CAD build for the part. Positions are in the model's coordinates, mm. Give positions to 0.01 mm unless a question says otherwise; leave off trailing zeros. Loops run counter-clockwise (first coordinate to the right, second up) from the corner with the lowest first, then second, coordinate; pieces in that order, holes last. Notation, with made-up numbers: (27, 60.25) -> (83, 60.25) arc R13 cw to (83, 78.25) -> close; hole circle Ø9 at (-14.75, -1.5). An arc over 180 degrees is marked (long way). Use one line per item in the form item = value.
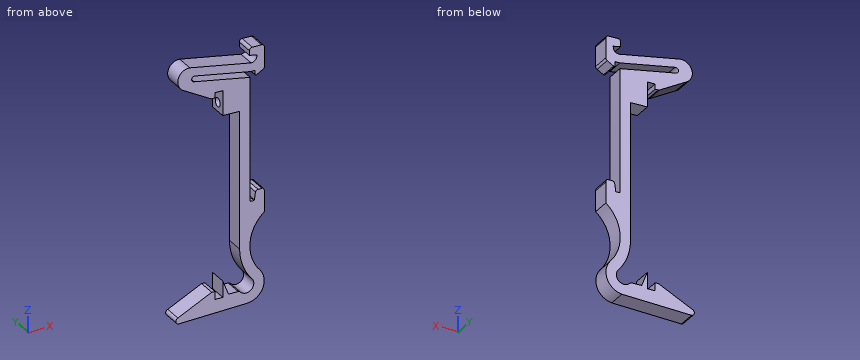
Autodesk Inventor part; units mm, degrees
ref_plane "YZ Plane" through (0, 0, 0) normal (1, 0, 0) x (0, 1, 0)
ref_plane "XZ Plane" through (0, 0, 0) normal (0, 1, 0) x (-1, 0, 0)
ref_plane "XY Plane" through (0, 0, 0) normal (0, 0, 1) x (1, 0, 0)
sketch "Sketch1" plane through (0, 0, 0) normal (0, 1, 0) x (-1, 0, 0)
  arc A0 (-159.7794, 702.6597) -> (-160.5669, 701.8721) centre (-159.7794, 701.8721) ccw
  line L0 (-155.7462, 702.6597) -> (-155.7462, 704.2667)
  line L1 (-155.7462, 704.2667) -> (-153.5139, 704.2667)
  line L2 (-153.5139, 704.2667) -> (-153.5139, 702.7873)
  line L3 (-153.5139, 702.7873) -> (-152.617, 702.7873)
  arc A1 (-164.1836, 648.4268) -> (-160.5669, 657.8731) centre (-174.7114, 657.8731) ccw
  line L4 (-160.5669, 657.8731) -> (-160.5669, 701.8721)
  arc A2 (-160.1794, 645.8656) -> (-160.7583, 645.6139) centre (-160.1783, 645.0714) ccw
  arc A3 (-164.1836, 648.4268) -> (-160.7583, 645.6139) centre (-162.4137, 647.0901) ccw
  line L5 (-155.7462, 648) -> (-155.7462, 645.3343)
  line L6 (-155.7462, 645.3343) -> (-153.4959, 645.3343)
  line L7 (-153.4959, 645.3343) -> (-153.4959, 647.6194)
  arc A4 (-143.0505, 641.0266) -> (-142.8499, 642.7649) centre (-143.1474, 641.9185) ccw
  line L8 (-163.0481, 641.9081) -> (-143.0505, 641.0266)
  arc A5 (-166.527, 650.2868) -> (-163.0481, 641.9081) centre (-162.4027, 647.0877) ccw
  arc A6 (-166.527, 650.2868) -> (-167.6435, 666.7468) centre (-174.834, 657.9912) ccw
  line L9 (-166.9993, 673.5601) -> (-165.874, 673.5549)
  arc A7 (-165.1258, 673.0171) -> (-165.874, 673.5549) centre (-165.8807, 672.7563) ccw
  arc A8 (-163.8545, 670.6656) -> (-163.5889, 670.9316) centre (-163.8582, 670.9349) ccw
  line L10 (-163.5889, 706.0242) -> (-163.5889, 706.0613)
  line L11 (-163.5889, 706.0613) -> (-147.5669, 708.9022)
  arc A9 (-147.5669, 708.9022) -> (-147.8271, 710.4852) centre (-147.6086, 709.7082) ccw
  line L12 (-147.8271, 710.4852) -> (-163.5899, 707.6952)
  line L13 (-163.5899, 707.6952) -> (-164.9831, 707.6944)
  line L14 (-164.9831, 707.6944) -> (-164.9826, 706.5463)
  arc A10 (-165.396, 706.3271) -> (-164.9826, 706.5463) centre (-165.2521, 706.5552) ccw
  line L15 (-165.396, 706.3271) -> (-167.2486, 707.3943)
  arc A11 (-167.6628, 708.0983) -> (-167.2486, 707.3943) centre (-166.8615, 708.0959) ccw
  line L16 (-167.6628, 708.0983) -> (-167.6658, 713.6939)
  arc A12 (-166.8627, 714.4991) -> (-167.6658, 713.6939) centre (-166.8611, 713.6943) ccw
  line L17 (-166.8627, 714.4991) -> (-164.1837, 714.5007)
  arc A13 (-163.3795, 713.6976) -> (-164.1837, 714.5007) centre (-164.1848, 713.6954) ccw
  line L18 (-163.3795, 713.6976) -> (-163.3787, 712.3581)
  line L19 (-163.3787, 712.3581) -> (-165.5216, 711.9789)
  line L20 (-165.5216, 711.9789) -> (-165.5215, 711.7106)
  arc A14 (-165.5215, 711.7106) -> (-163.8456, 710.1095) centre (-163.9177, 711.7116) ccw
  line L21 (-163.8456, 710.1095) -> (-146.318, 713.1891)
  arc A15 (-144.6103, 707.1134) -> (-146.318, 713.1891) centre (-146.0422, 709.9888) ccw
  arc A16 (-152.617, 702.7873) -> (-152.2474, 702.8795) centre (-152.6236, 703.6003) ccw
  line L22 (-155.7462, 702.6597) -> (-155.7462, 700.1597)
  line L23 (-155.7462, 700.1597) -> (-156.9462, 700.1597)
  line L24 (-156.9462, 700.1597) -> (-157.7628, 702.6597)
  line L25 (-157.7628, 702.6597) -> (-159.7794, 702.6597)
  line L26 (-155.7462, 648) -> (-155.7462, 650)
  line L27 (-155.7462, 650) -> (-157.3545, 645.8656)
  line L28 (-157.3545, 645.8656) -> (-160.1794, 645.8656)
  line L29 (-144.6103, 707.1134) -> (-152.2474, 702.8795)
  line L30 (-152.5619, 647.6194) -> (-153.4959, 647.6194)
  line L31 (-163.8545, 670.6656) -> (-164.6545, 670.6656)
  arc A17 (-164.8084, 670.8401) -> (-164.6545, 670.6656) centre (-164.6322, 670.8403) ccw
  line L32 (-163.5889, 670.9316) -> (-163.5889, 706.0613)
  line L33 (-164.8084, 670.8401) -> (-165.1258, 673.0171)
  line L34 (-167.6435, 666.7468) -> (-167.6666, 672.6833)
  line L35 (-166.9993, 673.5601) -> (-167.2486, 673.5601)
  arc A18 (-167.2486, 673.5601) -> (-167.6666, 672.6833) centre (-166.547, 672.6876) ccw
  line L36 (-142.8499, 642.7649) -> (-152.5619, 647.6194)
  point P0 (-160.5669, 683.588)
  dimension "d2" = 43.999
  dimension "d6" = 2.5
  dimension "d7" = 1.2
  dimension "d8" = 2
  dimension "d18" = 0.8
  dimension "d20" = 2.2
extrude "Extrusion1" add sketch "Sketch1" along normal blind 5.3
sketch "Sketch2" plane through (0, 0, 0) normal (0, -1, 0) x (1, 0, 0)
  line L0 (156.9462, 700.1597) -> (155.7462, 700.1597)
  line L1 (155.7462, 700.1597) -> (155.7462, 697.1597)
  line L2 (155.7462, 697.1597) -> (160.5669, 697.1597)
  line L3 (160.5669, 657.8731) -> (160.5669, 701.8721)
  line L4 (160.5669, 697.1597) -> (160.5783, 702.6397)
  line L5 (160.5783, 702.6397) -> (155.7462, 704.198)
  line L6 (155.7462, 704.198) -> (155.7462, 700.1597)
  point P0 (0, 0)
  dimension "d9" = 3
extrude "Extrusion2" add sketch "Sketch2" against normal blind 5.3
sketch "Sketch3" plane through (155.7462, 0, 704.2667) normal (-1, 0, 0) x (0, 0, 1)
  circle A0 centre (-4.5576, 2.65) radius 1.25
  line L0 (-7.107, 5.3) -> (0, 5.3)
  line L1 (0, 0) -> (-7.107, 0)
  point P0 (-704.2667, 0)
  dimension "d12" = 2.5
  dimension "d14" = 2.65
  dimension "d15" = 2.65
extrude "Extrusion3" cut sketch "Sketch3" against normal blind 5
properties part number "raspDinClipmmv3"
1. Cut at A-A, the plane z = 675.5. Write the cut outline in (x, y).
Result sheet:
outline = (160.57, 0) -> (163.59, 0) -> (163.59, 5.3) -> (160.57, 5.3) -> close
2. Cut at B-B, the plane z = 653. Write the cut outline in (x, y).
Result sheet:
outline = (161.43, 0) -> (164.66, 0) -> (164.66, 5.3) -> (161.43, 5.3) -> close
3. Drill centre lines: line 1 (Z direction, x = 160, y = 3.6); line 2 (Z direction, x = 154, y = 2.4); line 3 (Z direction, x = 158.25, y = 1.15). Where is each one in solid material? Low to high.
Result sheet:
line_1 = 641.77 to 645.87, 697.16 to 698.9, 700.52 to 706.7, 708.33 to 710.79
line_2 = 641.51 to 645.33, 704.27 to 707.76, 709.39 to 711.84
line_3 = 641.7 to 645.87, 697.16 to 707.01, 708.64 to 711.09
4. Drop flat-ended pins along their axis: P1, Ø1.5, axis at x = 160, y = 0.5, coming from the +Z side; P2, Ø2, axis at y = 2, z = 699.5, coming from the -X side; P3, Ø1.4, axis at y = 2.5, z = 648, coming from the -X side; P4, Ø2.5, axis at x = 147.61, z = 709.71, coming from the +Y side. Give the stop position or say it passes through.
Result sheet:
P1 = 710.92
P2 = 155.75
P3 = 151.92
P4 = 5.3
